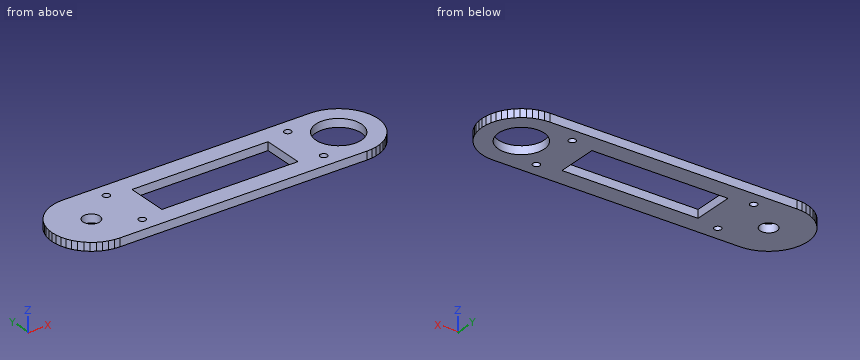
Solid Edge part; units mm, degrees
sketch "Sketch1" plane through (0, 0, 0) normal (0, 0, 1) x (1, 0, 0)
  line L0 (120, -19) -> (122.48, -18.8375)
  line L1 (122.48, -18.8375) -> (124.9176, -18.3526)
  line L2 (124.9176, -18.3526) -> (127.271, -17.5537)
  line L3 (127.271, -17.5537) -> (129.5, -16.4545)
  line L4 (129.5, -16.4545) -> (131.5665, -15.0737)
  line L5 (131.5665, -15.0737) -> (133.435, -13.435)
  line L6 (133.435, -13.435) -> (135.0737, -11.5665)
  line L7 (135.0737, -11.5665) -> (136.4545, -9.5)
  line L8 (136.4545, -9.5) -> (137.5537, -7.271)
  line L9 (137.5537, -7.271) -> (138.3526, -4.9176)
  line L10 (138.3526, -4.9176) -> (138.8375, -2.48)
  line L11 (138.8375, -2.48) -> (139, 0)
  line L12 (139, 0) -> (138.8375, 2.48)
  line L13 (138.8375, 2.48) -> (138.3526, 4.9176)
  line L14 (138.3526, 4.9176) -> (137.5537, 7.271)
  line L15 (137.5537, 7.271) -> (136.4545, 9.5)
  line L16 (136.4545, 9.5) -> (135.0737, 11.5665)
  line L17 (135.0737, 11.5665) -> (133.435, 13.435)
  line L18 (133.435, 13.435) -> (131.5665, 15.0737)
  line L19 (131.5665, 15.0737) -> (129.5, 16.4545)
  line L20 (129.5, 16.4545) -> (127.271, 17.5537)
  line L21 (127.271, 17.5537) -> (124.9176, 18.3526)
  line L22 (124.9176, 18.3526) -> (122.48, 18.8375)
  line L23 (122.48, 18.8375) -> (120, 19)
  line L24 (120, 19) -> (0, 19)
  line L25 (0, 19) -> (-2.48, 18.8375)
  line L26 (-2.48, 18.8375) -> (-4.9176, 18.3526)
  line L27 (-4.9176, 18.3526) -> (-7.271, 17.5537)
  line L28 (-7.271, 17.5537) -> (-9.5, 16.4545)
  line L29 (-9.5, 16.4545) -> (-11.5665, 15.0737)
  line L30 (-11.5665, 15.0737) -> (-13.435, 13.435)
  line L31 (-13.435, 13.435) -> (-15.0737, 11.5665)
  line L32 (-15.0737, 11.5665) -> (-16.4545, 9.5)
  line L33 (-16.4545, 9.5) -> (-17.5537, 7.271)
  line L34 (-17.5537, 7.271) -> (-18.3526, 4.9176)
  line L35 (-18.3526, 4.9176) -> (-18.8375, 2.48)
  line L36 (-18.8375, 2.48) -> (-19, 0)
  line L37 (-19, 0) -> (-18.8375, -2.48)
  line L38 (-18.8375, -2.48) -> (-18.3526, -4.9176)
  line L39 (-18.3526, -4.9176) -> (-17.5537, -7.271)
  line L40 (-17.5537, -7.271) -> (-16.4545, -9.5)
  line L41 (-16.4545, -9.5) -> (-15.0737, -11.5665)
  line L42 (-15.0737, -11.5665) -> (-13.435, -13.435)
  line L43 (-13.435, -13.435) -> (-11.5665, -15.0737)
  line L44 (-11.5665, -15.0737) -> (-9.5, -16.4545)
  line L45 (-9.5, -16.4545) -> (-7.271, -17.5537)
  line L46 (-7.271, -17.5537) -> (-4.9176, -18.3526)
  line L47 (-4.9176, -18.3526) -> (-2.48, -18.8375)
  line L48 (-2.48, -18.8375) -> (0, -19)
  line L49 (0, -19) -> (120, -19)
  circle A0 centre (0, 0) radius 4.1
  circle A1 centre (120, 0) radius 11.1
  line L50 (27, -10) -> (93, -10)
  line L51 (93, -10) -> (93, 10)
  line L52 (93, 10) -> (27, 10)
  line L53 (27, 10) -> (27, -10)
  circle A2 centre (16, -12) radius 1.7
  circle A3 centre (16, 12) radius 1.7
  circle A4 centre (104, -12) radius 1.7
  circle A5 centre (104, 12) radius 1.7
extrude "Protrusion1" add sketch "Sketch1" along normal blind 4
Design review of the part built by this model. Coordinates are the model's own, in mm. Give positions to 0.01 mm unless a question says otherwise; leave off trailing zeros. Write each loop counter-clockwise with the first axis right and the second up, starting at its lowest first coordinate (ties: lowest second). Pieces come first, ordered by that corner, then holes. Notation, with made-up numbers: M -8,53.5 L 11,53.5 A19 cw 11,61.5 Z; hole C 58.5,-9 d4. An arc over 180 degrees is marked long. Return JSON: item names as keys, results as strings. Group by question number.
Item 1: Clearance check with a flat-ended pin moving along its axis: pin 1 Ø2 at (y, z) = (2, 1) entering from +X. State where the tip first meets the part, or that it passes through.
Item 2: Wall thickness on line 1 along Y through (x, z) = (104, 2); line 2 along Y through (x, z) = (0, 2.05); line 3 along Y through (x, z) = (120, 2.75): over which ranges is each line inside the solid? List them lowest first.
Item 3: Take a section at B-B (z = 2.4). Count the separate pieces of the cut face and the enclosed holes in it, plus the area to 3 significant figures.
Item 4: Take a section at A-A (x = 89). Give the boundary of the cut face in (y, z).
Return value:
{
 "1": {"pin 1": "stops at x = 138.93"},
 "2": {"line 1": "y = -19 to -13.7, -10.3 to 10.3, 13.7 to 19", "line 2": "y = -19 to -4.1, 4.1 to 19", "line 3": "y = -19 to -11.1, 11.1 to 19"},
 "3": {"separate pieces": "1", "enclosed holes": "7", "area": "3,890 mm2"},
 "4": {"outline": "M -19,0 L -10,0 L -10,4 L -19,4 Z; M 10,0 L 19,0 L 19,4 L 10,4 Z"}
}
